```python
from build123d import *

# Parameters (mm, degrees)
F1_DEPTH = 25


with BuildPart() as f1:
    # F0 (on Front) → F1 (new body)
    with BuildSketch(Plane.XZ):
        with BuildLine():
            ThreePointArc((-28.190229, 45.313943), (-24.214198, 42.800089), (-22.182589, 38.557349))
            ThreePointArc((-22.182589, 38.557349), (0.896682, -44.473951), (20.610411, 39.420139))
            ThreePointArc((20.610411, 39.420139), (22.279856, 43.485217), (26.273011, 45.320053))
            ThreePointArc((26.273011, 45.320053), (22.742729, 68.079793), (3.432866, 80.633594))
            Line((3.432866, 80.633594), (3.432866, 99.945173))
            ThreePointArc((3.432866, 99.945173), (1.716433, 101.661606), (0, 99.945173))
            Line((0, 99.945173), (0, 80.961105))
            ThreePointArc((0, 80.961105), (-1.559237, 80.971042), (-3.116643, 80.894866))
            Line((-3.116643, 80.894866), (-3.116643, 87.447404))
            ThreePointArc((-3.116643, 87.447404), (-5.188906, 89.519667), (-7.26117, 87.447404))
            Line((-7.26117, 87.447404), (-7.26117, 80.265008))
            ThreePointArc((-7.26117, 80.265008), (-25.177238, 67.251534), (-28.190229, 45.313943))
        make_face()
        with BuildLine():
            ThreePointArc((-27.778708, 45.710137), (-24.574012, 67.281705), (-6.76117, 79.863648))
            Line((-6.76117, 79.863648), (-6.76117, 87.447404))
            ThreePointArc((-6.76117, 87.447404), (-5.188906, 89.019667), (-3.616643, 87.447404))
            Line((-3.616643, 87.447404), (-3.616643, 80.349799))
            ThreePointArc((-3.616643, 80.349799), (-1.559979, 80.470911), (0.5, 80.438979))
            Line((0.5, 80.438979), (0.5, 99.945173))
            ThreePointArc((0.5, 99.945173), (1.716433, 101.161606), (2.932866, 99.945173))
            Line((2.932866, 99.945173), (2.932866, 80.202862))
            ThreePointArc((2.932866, 80.202862), (22.110002, 68.132408), (25.88031, 45.788658))
            ThreePointArc((25.88031, 45.788658), (21.690506, 43.580432), (20.113465, 39.1146))
            ThreePointArc((20.113465, 39.1146), (0.866103, -43.974461), (-21.63804, 38.292279))
            ThreePointArc((-21.63804, 38.292279), (-23.633494, 42.891018), (-27.778708, 45.710137))
        make_face(mode=Mode.SUBTRACT)
    extrude(amount=F1_DEPTH)


solid = f1.part
```
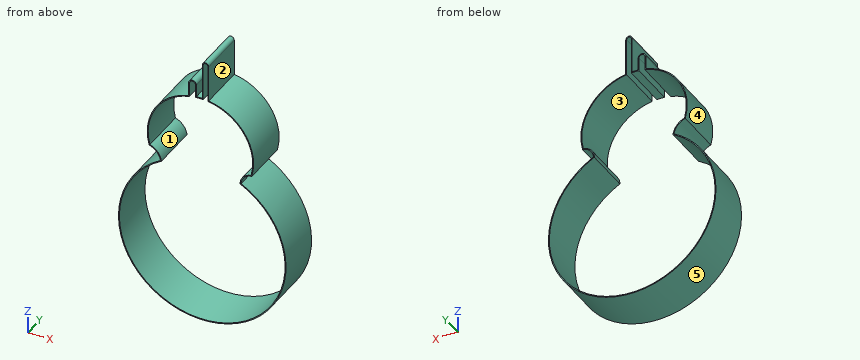
Source: CAD feature listing. Evaluate the final solid. Frame: model axes, mm. Face numbers are marked on the shaded views. A direction names the side the tool comes from. Round coordinates to 2 decimals unless told otherwise and drop trailing zeros. Loops run counter-clockwise (first coordinate to the right, second up) from the corner with the lowest first, then second, coordinate; pieces in that order, holes last. Notation, with made-up numbers: M 5.25,-28.75 L 28.25,-28.75 A13 cw 28.25,-12.75 Z; hole C 2,-34 d11. An arc over 180 degrees is marked long. Use a Markdown table: item, result. Add a question column.
1. Ray query, line 1 along X through (y, z) = (-15, 83); line 2 along X through (y, z) = (-18.5, 0); line 3 along X through (y, z) = (-6.5, 67.5). Return the intervals inside material, ascending. Write a range as [from, to].
2. Cut plane B-B, the plane x = 22. Output: boundary loops of the cut face in (y, z), and give its area (3 significant figures).
3. Cut plane C-C, the plane x = 34.5. Output: boundary loops of the cut face in (y, z).
4. Contact query for flat-ended pins moving along their axis: pin 1 (6 mm diameter, centred on y = -15.5, z = 94, fed in from -X); pin 2 (1.5 mm diameter, centred on x = -9, y = -21.5, fed in from +Z); pin 3 (4 mm diameter, centred on y = -3, z = 41.5, fed in from -X). Output: stop coordinate, or through.
5. Pull-direction query (X, two-part tool) for the marked faces 3, 4 and 5; classes: +X half, -X half, draft (parallel to the pull), parting line (faces both ways), or undercut.
6. Cut plane D-D, the plane y = -12. Output: boundary loops of the cut face in (x, z) (1 decimal), and give its area (3 significant figures).
7. Cut plane A-A, the plane z = 0. Output: boundary loops of the cut face in (x, y), and give its area (3 significant figures).
8. Set-up query: the marked faces 1 and 2. Return all of +Z, -Z, +X, -X, +Y, -Y with unobstructed straight access to the full face (end or side cutting, diameter ignored); none if empty.
Solution:
| question | item | result |
|---|---|---|
| 1 | line 1 | x = [-7.26, -6.76], [-3.62, -3.12], [0, 0.5], [2.93, 3.43] |
| 1 | line 2 | x = [-44.48, -43.98], [43.98, 44.48] |
| 1 | line 3 | x = [-25.03, -24.44], [22.52, 23.11] |
| 2 | outline | M -25,-38.66 L 0,-38.66 L 0,-38.09 L -25,-38.09 Z; M -25,38.09 L 0,38.09 L 0,38.66 L -25,38.66 Z; M -25,43.17 L 0,43.17 L 0,43.91 L -25,43.91 Z; M -25,68.3 L 0,68.3 L 0,69.17 L -25,69.17 Z |
| 2 | area | 69.2 mm2 |
| 3 | outline | M -25,-28.08 L 0,-28.08 L 0,-27.28 L -25,-27.28 Z; M -25,27.28 L 0,27.28 L 0,28.08 L -25,28.08 Z |
| 4 | pin 1 | stops at x = 0 |
| 4 | pin 2 | stops at z = 80.02 |
| 4 | pin 3 | stops at x = -24.91 |
| 5 | face 3 | undercut |
| 5 | face 4 | -X half |
| 5 | face 5 | parting line |
| 6 | outline | M -28.2,45.3 A8.5 cw -22.2,38.6 A44.5 ccw long 20.6,39.4 A6 cw 26.3,45.3 A28.2 ccw 3.4,80.6 L 3.4,99.9 A1.7 ccw 0,99.9 L 0,81 A28.2 ccw -3.1,80.9 L -3.1,87.4 A2.1 ccw -7.3,87.4 L -7.3,80.3 A28.2 ccw Z; hole M -27.8,45.7 A9 cw -21.6,38.3 A44 ccw long 20.1,39.1 A6.5 cw 25.9,45.8 A27.7 ccw 2.9,80.2 L 2.9,99.9 A1.2 ccw 0.5,99.9 L 0.5,80.4 A27.7 ccw -3.6,80.3 L -3.6,87.4 A1.6 ccw -6.8,87.4 L -6.8,79.9 A27.7 ccw Z |
| 6 | area | 206 mm2 |
| 7 | outline | M -44.48,-25 L -43.98,-25 L -43.98,0 L -44.48,0 Z; M 43.98,-25 L 44.48,-25 L 44.48,0 L 43.98,0 Z |
| 7 | area | 25.0 mm2 |
| 8 | face 1 | +Y, -Y |
| 8 | face 2 | +Z, +X, +Y, -Y |
